Read the model definition and answer for the solid it produces. Units are mm, in the model's axes. A direction names the side the tool comes from. Round coordinates to 2 decimals unless told otherwise and drop trailing zeros. Order: outer loops, then holes, each group sorted by start corner. A loop starts at its lowest first (then second) coordinate and runs counter-clockwise, first axis right, second up. Notation, with made-up numbers: (-23.75, 8.5) -> (-13.75, 8.5) arc R24 cw to (-13.75, 28.5) -> close; hole circle Ø1 at (4.25, 50.25). An arc over 180 degrees is marked (long way). Answer as a JSON object with one key per item and string values. Group by question number.
Item 1: For faces 4 (the cylindrical face through (10.7, 3.45, 4.33)), 5 (the flat face through (9, 7, 4)), determine the directions among +Z, -Z, +X, -X, +Y, -Y from which every point of the face is accessible in a straight line to the end or side of a thin tool.
Item 2: Section D-D, the plane z = -11.5 is taken. Write down the section's boundary in (x, y).
Item 3: Given P1, Ø6, axis at x = 0, z = -11.5, coming from the +Y side; P2, Ø4, axis at y = 7, z = 5, coming from the -X side; P3, Ø1, axis at x = -5.5, z = 2, coming from the +Y side; P4, Ø9, axis at x = 0, z = 0, coming from the -Y side, each flat-ended and moving along its own axis, determine where each tip first touches the part or whether it passes through.
Item 4: Section A-A, the plane z = 0 is taken. Write down the section's boundary in (x, y), plus the area to 3 significant figures.
Item 5: Section B-B, the plane x = 0 is taken. Write down the section's boundary in (y, z), plus the area to 3 significant figures.
Item 6: The mould has two halves that part along Z. Classify faces 1 (the cylindrical face through (-11.459, 8.521, 2.867)), 2 (the cylindrical face through (-14.985, 4.93, -0.66)), 3 (the flat face through (6, 0, 0)): pulls with the +Z half, pulls with the -Z half, needs draft (parallel to the pull), parting line crosses it, or undercut.
Item 7: Section C-C, the plane y = 2.5 is taken. Write down the section's boundary in (x, z).
Item 8: Consider probe 1 along Z at (x, y) = (0, 2); probe 2 along X at (y, z) = (3.5, 0); probe 3 along X at (y, z) = (8.5, 6.5). Determine where each line is inside the solid, lowest interval first. Write a range as from..to.
from build123d import *

# Parameters (mm, degrees)
SKETCH1_R                      = 15
SKETCH1_R_2                    = 5.5
BOSS_EXTRUDE1_DEPTH            = 10
FILLET1_R                      = 3
CBORE_FOR_M3_SHCS1_D           = 3.2
CBORE_FOR_M3_SHCS1_CBORE_D     = 6.5
CBORE_FOR_M3_SHCS1_CBORE_DEPTH = 3
CIRPATTERN1_COUNT              = 3


with BuildPart() as part:
    # Sketch1 → Boss-Extrude1 (new body)
    with BuildSketch(Plane(origin=(0, 0, 0), x_dir=(1, 0, 0), z_dir=(0, 1, 0))):
        Circle(SKETCH1_R)
        Circle(SKETCH1_R_2, mode=Mode.SUBTRACT)
    extrude(amount=BOSS_EXTRUDE1_DEPTH)

    # Fillet1
    fillet1_edges = [part.edges().sort_by_distance(p)[0] for p in [
        (-5.5, 10, 0),
    ]]
    fillet(fillet1_edges, radius=FILLET1_R)

    # CBORE for M3 SHCS1 (through all)
    with Locations(Plane(origin=(0, 10, 0), x_dir=(-1, 0, 0), z_dir=(0, 1, 0))):
        with Locations((0, -11.5)):
            cbore_for_m3_shcs1 = CounterBoreHole(CBORE_FOR_M3_SHCS1_D / 2, CBORE_FOR_M3_SHCS1_CBORE_D / 2, CBORE_FOR_M3_SHCS1_CBORE_DEPTH)

    # CirPattern1: CBORE for M3 SHCS1 ×3 about axis
    cirpattern1_axis = Axis((0, 0, 0), (0, 1, 0))
    for i in range(1, CIRPATTERN1_COUNT):
        add(cbore_for_m3_shcs1.rotate(cirpattern1_axis, i * 360 / CIRPATTERN1_COUNT), mode=Mode.SUBTRACT)


solid = part.part
Values found:
{
 "1": {"face 4": "+Y, -Y", "face 5": "+Y"},
 "2": {"outline": "(-9.63, 0) -> (-1.6, 0) -> (-1.6, 7) -> (-3.25, 7) -> (-3.25, 10) -> (-9.63, 10) -> close; (1.6, 0) -> (9.63, 0) -> (9.63, 10) -> (3.25, 10) -> (3.25, 7) -> (1.6, 7) -> close"},
 "3": {"P1": "y = 7", "P2": "x = -14.7", "P3": "y = 9.09", "P4": "through"},
 "4": {"outline": "(-15, 0) -> (-5.5, 0) -> (-5.5, 7) arc R3 ccw to (-8.5, 10) -> (-15, 10) -> close; (5.5, 0) -> (15, 0) -> (15, 10) -> (8.5, 10) arc R3 ccw to (5.5, 7) -> close", "area": "186 mm2"},
 "5": {"outline": "(0, -15) -> (10, -15) -> (10, -14.75) -> (7, -14.75) -> (7, -13.1) -> (0, -13.1) -> close; (0, -9.9) -> (7, -9.9) -> (7, -8.25) -> (9.99, -8.25) arc R3 ccw to (7, -5.5) -> (0, -5.5) -> close; (0, 5.5) -> (7, 5.5) arc R3 ccw to (10, 8.5) -> (10, 15) -> (0, 15) -> close", "area": "144 mm2"},
 "6": {"face 1": "undercut", "face 2": "parting line crosses it", "face 3": "needs draft"},
 "7": {"outline": "circle Ø30 at (0, 0); hole circle Ø3.2 at (-9.96, 5.75); hole circle Ø11 at (0, 0); hole circle Ø3.2 at (0, -11.5); hole circle Ø3.2 at (9.96, 5.75)"},
 "8": {"probe 1": "-15..-13.1, -9.9..-5.5, 5.5..15", "probe 2": "-15..-5.5, 5.5..15", "probe 3": "-13.52..-13.12, -6.8..6.8, 13.12..13.52"}
}
